```python
from build123d import *

# Parameters (mm, degrees)
F0_W      = 60
F0_H      = 40
F1_DEPTH  = 40
F3_DEPTH  = 30
F6_DEPTH  = 25
F4_W      = 10
F4_H      = 30
F7_DEPTH  = 25
F10_DEPTH = 25
F8_W      = 10
F8_H      = 30
F11_DEPTH = 25


with BuildPart() as f1:
    # F0 (on Front) → F1 (new body)
    with BuildSketch(Plane.XZ):
        with Locations((30, 20)):
            Rectangle(F0_W, F0_H)
    extrude(amount=F1_DEPTH)

    # F2 (on face) → F3 (cut)
    with BuildSketch(Plane.XY.offset(40)):
        Polygon((40, 0), (20, 0), (10, -40), (50, -40), align=None)
    extrude(amount=-F3_DEPTH, mode=Mode.SUBTRACT)

    # F5 (on face) → F6 (cut)
    with BuildSketch(Plane(origin=(0, 0, 0), x_dir=(0, -1, 0), z_dir=(-1, 0, 0))):
        Polygon((40, 40), (0, 40), (40, 9.9955964833), align=None)
    extrude(amount=-F6_DEPTH, mode=Mode.SUBTRACT)

    # F4 (on face) → F7 (cut)
    with BuildSketch(Plane.XZ.offset(40)):
        with Locations((5, 25)):
            Rectangle(F4_W, F4_H)
    extrude(amount=F7_DEPTH, mode=Mode.SUBTRACT)

    # F9 (on face) → F10 (cut)
    with BuildSketch(Plane.YZ.offset(60)):
        Polygon((-40, 10.0021371618), (0, 40), (-40, 40), align=None)
    extrude(amount=-F10_DEPTH, mode=Mode.SUBTRACT)

    # F8 (on face) → F11 (cut)
    with BuildSketch(Plane.XZ.offset(40)):
        with Locations((55, 25)):
            Rectangle(F8_W, F8_H)
    extrude(amount=F11_DEPTH, mode=Mode.SUBTRACT)


solid = f1.part
```
For this review, take the finished solid that the model builds, in its own axes (mm). A direction names the side the tool comes from. Coordinates: 2 decimals unless noted, no trailing zeros. Loops run counter-clockwise (first coordinate to the right, second up) from the corner with the lowest first, then second, coordinate; pieces in that order, holes last.
1. Add section D-D, the plane z = 36. Give the boundary of the cut face in (x, y), then the cut area to 3 significant figures.
2. Add section B-B, the plane y = -32.5. Give the boundary of the cut face in (x, z) (3 decimals), then the cut area to 3 significant figures.
3. For line 1 (X direction, y = -24.5, z = 12) (3 decimals); line 2 (X direction, y = -10, z = 27.5); line 3 (Z direction, x = 36, y = -17.5), list the stretches that pass through material, from the lowest coordinate up.
4. Add section A-A, the plane z = 17.5. Give the boundary of the cut face in (x, y).
5. For faces 1 (the flat face through (17.3, -10.8, 18.5)), 2 (the flat face through (30, -40, 5)), list the 3-axis set-ups (+Z, -Z, +X, -X, +Y, -Y) from which the entire face can be reached by the end or side of a thin tool; tool diameter is ignored.
6. Mouldability with a two-part tool opening along Y and no side actions: class faces 3 (the flat face through (42.848, -11.391, 18.543)), 4 (the flat face through (0, -15, 15)), 5 (the flat face through (30, 0, 7)) as +Y half, -Y half, draft (parallel to the pull), parting line (faces both ways), or undercut.
7. Insertion check: P1, Ø1.5, axis at x = 28, y = -30, coming from the +Z side. The pin has a flat end and moves straight along its axis. Give the tip position at first contact, or say it passes through.
Result:
1. outline: (0, -5.33) - (18.67, -5.33) - (20, 0) - (0, 0) - close; (40, 0) - (41.33, -5.33) - (60, -5.33) - (60, 0) - close
1. area: 206 mm2
2. outline: (0, 0) - (60, 0) - (60, 15.627) - (48.125, 15.627) - (48.125, 10) - (11.875, 10) - (11.875, 15.621) - (0, 15.621) - close
2. area: 734 mm2
3. line 1: x = 0 to 13.875, 46.125 to 60
3. line 2: x = 0 to 17.5, 42.5 to 60
3. line 3: z = 0 to 10
4. outline: (0, -30) - (12.5, -30) - (20, 0) - (0, 0) - close; (40, 0) - (47.5, -30) - (60, -30) - (60, 0) - close
5. face 1: +Z, -Y
5. face 2: +Z, -Z, +X, -X, -Y
6. face 3: -Y half
6. face 4: draft
6. face 5: +Y half
7. P1: stops at z = 10
